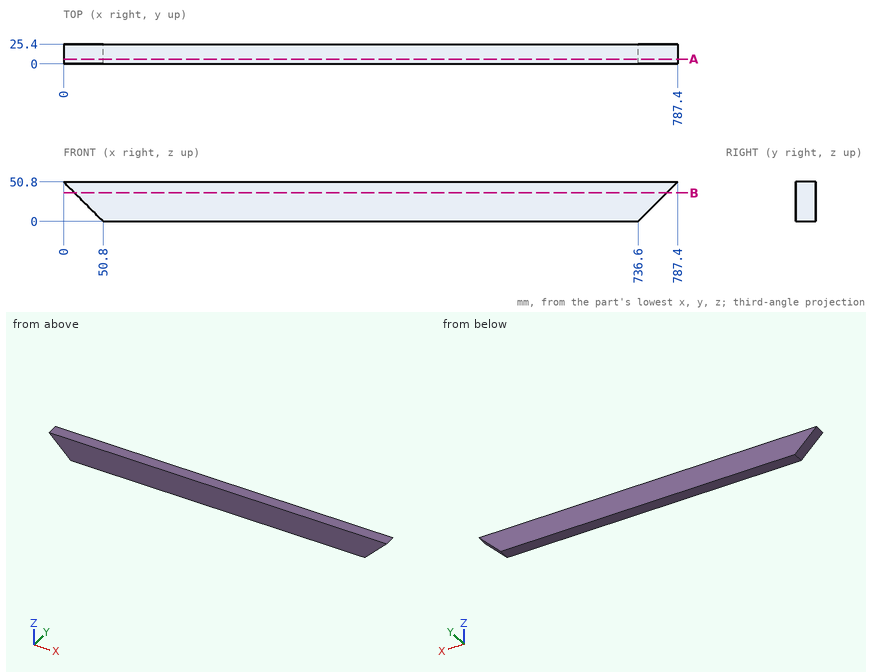
Source: three-view drawing plus pictorial views. Frame: mm from the lowest corner of the part. Give positions to 0.01 mm unless a question says otherwise; leave off trailing zeros. Order: outer loops, then holes, each group sorted by start corner. A loop starts at its lowest first (then second) coordinate and runs counter-clockwise, first axis right, second up. Notation, with made-up numbers: (8, 85.5) - (44, 85.5) arc R18 ccw to (44, 97.5) - close; hole circle Ø2 at (-22.75, -0.5). An arc over 180 degrees is marked (long way). Put each result on its own line as item: value.
Item 1: Section query B-B, the plane z = 36.5. Return loops of the section in (x, y).
Found:
outline: (14.3, 0) - (773.1, 0) - (773.1, 25.4) - (14.3, 25.4) - close
Item 2: Section query A-A, the plane y = 6. Return loops of the section in (x, z).
Found:
outline: (0, 50.8) - (50.8, 0) - (736.6, 0) - (787.4, 50.8) - close
Item 3: Contact query for a flat-ended pin moving along its axis: pin 1 (1.5 mm diameter, centred on y = 3.5, z = 39, fed in from +X). Output: stop coordinate, or through.
Found:
pin 1: stops at x = 776.35
Item 4: Ray query, L1, parallel to X at y = 5.5, z = 24; L2, parallel to X at y = 19, z = 16.5; L3, parallel to Z at x = 50, y = 24. Return the intervals inside material, ascending. Write a range as from..to.
Found:
L1: x = 26.8..760.6
L2: x = 34.3..753.1
L3: z = 0.8..50.8
